```python
from build123d import *

# Parameters (mm, degrees)
SKETCH1_W            = 45
SKETCH1_H            = 290
BOSS_EXTRUDE1_DEPTH  = 4
M5_CLEARANCE_HOLE1_D = 5.3
FILLET1_R            = 1


with BuildPart() as part:
    # Sketch1 → Boss-Extrude1 (new body)
    with BuildSketch(Plane.XY):
        with Locations((0, 5)):
            Rectangle(SKETCH1_W, SKETCH1_H)
    extrude(amount=BOSS_EXTRUDE1_DEPTH)

    # M5 Clearance Hole1 (through all)
    with Locations(Plane.XY.offset(4)):
        with Locations((-16, 142.5), (-16, 112.5), (-16, -102.5), (-16, -132.5), (16, -132.5), (16, -102.5), (16, 112.5), (16, 142.5), (-16, 30), (-16, 0), (16, 0), (16, 30), (-16, 90), (-16, 60), (-16, -50), (-16, -80), (16, -80), (16, -50), (16, 60), (16, 90)):
            Hole(M5_CLEARANCE_HOLE1_D / 2)

    # Fillet1
    fillet1_edges = [part.edges().sort_by_distance(p)[0] for p in [
        (-22.5, 150, 2),
        (22.5, 150, 2),
        (22.5, -140, 2),
        (-22.5, -140, 2),
    ]]
    fillet(fillet1_edges, radius=FILLET1_R)


solid = part.part
```
Design review of the part built by this model. Coordinates are the model's own, in mm. Coordinates: 2 decimals unless noted, no trailing zeros. Order: outer loops, then holes, each group sorted by start corner. A loop starts at its lowest first (then second) coordinate and runs counter-clockwise, first axis right, second up. Notation, with made-up numbers: (3.5, -20) - (29.5, -20) arc R28 ccw to (29.5, 0) - close; hole circle Ø4 at (44.25, 59). An arc over 180 degrees is marked (long way). Answer in a Markdown table with one row per item.
(1) Consider section B-B on y = -50. State the section outline as (x, z) points.
Checked values:
| item | result |
|---|---|
| outline | (-22.5, 0) - (-18.65, 0) - (-18.65, 4) - (-22.5, 4) - close; (-13.35, 0) - (13.35, 0) - (13.35, 4) - (-13.35, 4) - close; (18.65, 0) - (22.5, 0) - (22.5, 4) - (18.65, 4) - close |
(2) Wall thickness on line 1 along X through (y, z) = (-132.5, 1.7); line 2 along X through (y, z) = (59, 1.3): over which ranges is each line inside the solid? List them lowest first. Write a range as from..to.
Checked values:
| item | result |
|---|---|
| line 1 | -22.5..-18.65, -13.35..13.35, 18.65..22.5 |
| line 2 | -22.5..-18.45, -13.55..13.55, 18.45..22.5 |
(3) Clearance check with flat-ended pins moving along their axes: pin 1 (5 mm diameter, centred on x = -16, y = 112.5, fed in from -Z); pin 2 (7 mm diameter, centred on x = -16, y = -132.5, fed in from -Z). State where each tip first meets the part, or that it passes through.
Checked values:
| item | result |
|---|---|
| pin 1 | through |
| pin 2 | z = 0 |
(4) The part is to be moulded in two halves that separate along Y. For faces 1 (the cylindrical face through (-18.45, -133.51, 1.97)), 2 (the flat face through (0, 7, 0)), say which applies: released by +Y, released by -Y, zero draft, split by the parting line, or undercut.
Checked values:
| item | result |
|---|---|
| face 1 | undercut |
| face 2 | zero draft |
(5) Consider section A-A on z = 3. Give the number of separate pieces and of enclosed holes in the cut face, plus the area to 3 significant figures.
Checked values:
| item | result |
|---|---|
| separate pieces | 1 |
| enclosed holes | 20 |
| area | 12,600 mm^2 |
